Part model, mm, in its own coordinate system. A direction names the side the tool comes from. Coordinates: 2 decimals unless noted, no trailing zeros. Order: outer loops, then holes, each group sorted by start corner. A loop starts at its lowest first (then second) coordinate and runs counter-clockwise, first axis right, second up.
1) Cut at A-A (z = -3). List the corners of the cut face in (x, y), and give its area (3 significant figures).
2) Cut at D-D (z = 4). List the corners of the cut face in (x, y), and give its area (3 significant figures).
3) Wall check: L1, parallel to X at y = -2.75, z = -3; L2, parallel to Z at x = 0, y = 27; L3, parallel to X at y = -6.25, z = -3. Give the ranges that are in metal, low to high.
4) Cut at C-C (y = 2). List the corners of the cut face in (x, z).
5) Cut at B-B (x = 0). List the corners of the cut face in (y, z), and give its area (3 significant figures).
6) Tool access for faces 1 (the flat face through (12.5, -5, -3)), 2 (the flat face through (9.4, 0, -1.6)), 3 (the cylindrical face through (0.65, 28.03, 1.07)), 4 (the flat face through (4.762, -1, 2)): list every direction of +Z, -Z, +X, -X, +Y, -Y with a clear straight run to the whole face (end or side of a thin tool).
7) Pin check, flat tips, straight feed: pin 1 Ø8 at (x, y) = (15.5, -24) entering from -Z; pin 2 Ø4 at (x, z) = (-13, -1) entering from +Y; pin 3 Ø5 at (x, z) = (-1, 3.5) entering from +Y. Stop position of each tip, or through.
8) Mould opens along X. For faces 5 (the flat face through (-12.5, -5, -3)), 6 (the flat face through (0, -6, 8)), 7 (the flat face through (0, 4.762, 4)) say: +X half, -X half, draft (parallel to the pull), parting line (faces both ways), or undercut.
Autodesk Inventor part; units mm, degrees
ref_plane "Work Plane1" through (0, 30, 0) normal (0, 1, 0) x (-1, 0, 0)
ref_plane "YZ Plane" through (0, 0, 0) normal (1, 0, 0) x (0, 1, 0)
ref_plane "XZ Plane" through (0, 0, 0) normal (0, 1, 0) x (-1, 0, 0)
sketch "Sketch1" plane through (0, 0, 0) normal (0, 0, 1) x (1, 0, 0)
  circle A0 centre (0, 0) radius 30
  line L0 (4.7625, -4.7625) -> (-4.7625, -4.7625)
  line L1 (-4.7625, -4.7625) -> (-4.7625, 4.7625)
  line L2 (-4.7625, 4.7625) -> (4.7625, 4.7625)
  line L3 (4.7625, 4.7625) -> (4.7625, -4.7625)
  line L4 (4.7625, -4.7625) -> (-4.7625, 4.7625) construction
  line L5 (-4.7625, -4.7625) -> (4.7625, 4.7625) construction
  dimension "d0" = 60
  dimension "d15" = 9.525
extrude "Extrusion1" add sketch "Sketch1" along normal blind 8
sketch "Sketch2" plane through (0, 0, 8) normal (0, 0, 1) x (1, 0, 0)
  circle A0 centre (0, 0) radius 30
  line L0 (0, 0) -> (0, 25) construction
  circle A1 centre (0, 25) radius 3
  dimension "d4" = 6
  dimension "d5" = 25
extrude "Extrusion2" [suppressed]
sketch "Sketch3" plane through (0, 0, 0) normal (0, 0, -1) x (-1, 0, 0)
  line L0 (-4.7625, 0) -> (-12.5, 0)
  line L1 (-12.5, 0) -> (-12.5, -10)
  line L2 (-12.5, -10) -> (12.5, -10)
  line L3 (12.5, -10) -> (12.5, 0)
  line L4 (12.5, 0) -> (4.7625, 0)
  line L5 (4.7625, 4.7625) -> (4.7625, -4.7625) construction
  line L6 (-4.7625, -4.7625) -> (-4.7625, 4.7625) construction
  line L7 (4.7625, -4.7625) -> (-4.7625, -4.7625) construction
  line L8 (4.7625, -4.7625) -> (4.7625, 4.7625)
  line L9 (4.7625, 0) -> (4.7625, -4.7625)
  line L10 (4.7625, -4.7625) -> (-4.7625, -4.7625)
  line L11 (-4.7625, 4.7625) -> (-4.7625, -4.7625)
  line L12 (-4.7625, -4.7625) -> (-4.7625, 0)
  dimension "d8" = 10
  dimension "d9" = 25
extrude "Extrusion3" add sketch "Sketch3" along normal blind 6
sketch "Sketch4" plane through (-12.5, 0, 0) normal (0, 1, 0) x (1, 0, 0)
  line L0 (21.1313, 6) -> (21.1313, 0) construction
  line L1 (3.8687, 6) -> (3.8687, 0) construction
  circle A0 centre (21.1312, 3) radius 1.4
  circle A1 centre (3.8687, 3) radius 1.4
  line L2 (7.7375, 0) -> (0, 0) construction
  line L3 (7.7375, 0) -> (7.7375, 6) construction
  line L4 (0, 6) -> (7.7375, 6) construction
  line L5 (0, 0) -> (0, 6) construction
  line L6 (25, 0) -> (17.2625, 0) construction
  line L7 (25, 0) -> (25, 6) construction
  line L8 (17.2625, 6) -> (25, 6) construction
  line L9 (17.2625, 0) -> (17.2625, 6) construction
  line L10 (0, 6) -> (7.7375, 6) construction
  line L11 (7.7375, 0) -> (0, 0) construction
  line L12 (17.2625, 6) -> (25, 6) construction
  dimension "d12" = 2.8
extrude "Extrusion4" cut sketch "Sketch4" against normal through all
ref_plane "Work Plane1" through (0, 30, 0) normal (0, 1, 0) x (-1, 0, 0)
sketch "Sketch5" plane through (0, 30, 0) normal (0, 1, 0) x (-1, 0, 0)
  line L0 (30, 8) -> (-30, 8) construction
  line L1 (-30, 0) -> (30, 0) construction
  line L2 (30, 8) -> (-30, 8) construction
  line L3 (0, 8) -> (0, 0) construction
  circle A0 centre (0, 4) radius 3
  dimension "d16" = 6
extrude "Extrusion5" cut sketch "Sketch5" against normal blind 4
properties part number "sensor wheel"
Geometry check:
1. outline: (-12.5, -10) - (-10.03, -10) - (-10.03, 0) - (-12.5, 0) - close; (-7.23, -10) - (7.23, -10) - (7.23, 0) - (4.76, 0) - (4.76, -4.76) - (-4.76, -4.76) - (-4.76, 0) - (-7.23, 0) - close; (10.03, -10) - (12.5, -10) - (12.5, 0) - (10.03, 0) - close
1. area: 149 mm2
2. outline: (-3, 26) - (-3, 29.85) arc R30 ccw (long way) to (3, 29.85) - (3, 26) - close; hole (-4.76, -4.76) - (4.76, -4.76) - (4.76, 4.76) - (-4.76, 4.76) - close
2. area: 2,710 mm2
3. L1: x = -12.5 to -10.03, -7.23 to -4.76, 4.76 to 7.23, 10.03 to 12.5
3. L2: z = 0 to 1, 7 to 8
3. L3: x = -12.5 to -10.03, -7.23 to 7.23, 10.03 to 12.5
4. outline: (-29.93, 0) - (-4.76, 0) - (-4.76, 8) - (-29.93, 8) - close; (4.76, 0) - (29.93, 0) - (29.93, 8) - (4.76, 8) - close
5. outline: (-30, 0) - (-10, 0) - (-10, -6) - (-4.76, -6) - (-4.76, 8) - (-30, 8) - close; (4.76, 0) - (30, 0) - (30, 1) - (26, 1) - (26, 7) - (30, 7) - (30, 8) - (4.76, 8) - close
5. area: 411 mm2
6. face 1: -Z, +X, +Y, -Y
6. face 2: -Z, +X, -X, +Y
6. face 3: +Y
6. face 4: +Z, -Z
7. pin 1: stops at z = 0
7. pin 2: stops at y = 27.8
7. pin 3: stops at y = 30
8. face 5: -X half
8. face 6: draft
8. face 7: undercut
